Geometry: final body of the model. Coordinates: model frame, mm. Face numbers are marked on the shaded views. A direction names the side the tool comes from. Give positions to 0.01 mm unless a question says otherwise; leave off trailing zeros. Order: outer loops, then holes, each group sorted by start corner. A loop starts at its lowest first (then second) coordinate and runs counter-clockwise, first axis right, second up. Notation, with made-up numbers: M 89.25,75 L 129.25,75 A24 ccw 129.25,105 Z; hole C 18,-3 d9. An arc over 180 degrees is marked long. Use CSV: the item, a comma, the result in double quotes.
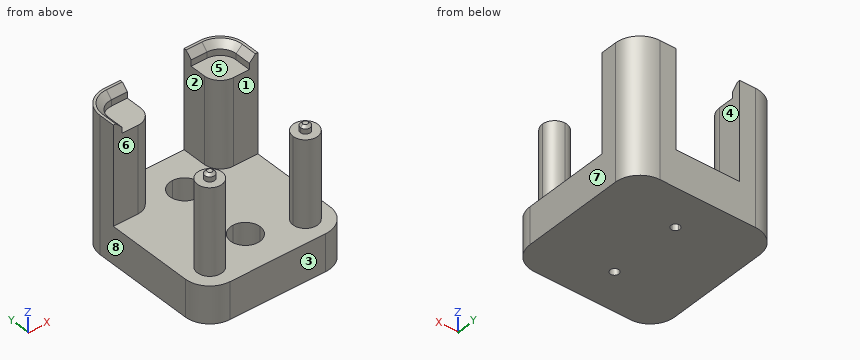
```python
from build123d import *

# Parameters (mm, degrees)
F0_W     = 26
F0_H     = 3.5
F1_DEPTH = 15
F2_DEPTH = 50
F3_DEPTH = 53
F4_DEPTH = 3
F5_DEPTH = 55
F6_SIZE  = 2.5
F7_SIZE  = 1


# Not quite as in the source:
# - a feature names something its author has since deleted; it is built from what else it names


with BuildPart() as f1:
    # F0 (on Top) → F1 (new body)
    with BuildSketch(Plane.XY):
        with Locations((0, 29.25)):
            Rectangle(F0_W, F0_H)
        with BuildLine():
            Line((29.5, -21), (29.5, 14.5))
            Line((29.5, 14.5), (26, 14.5))
            Line((26, 14.5), (19.5, 14.5))
            Line((19.5, 14.5), (19.5, 0))
            Line((19.5, 0), (19.5, -16))
            ThreePointArc((19.5, -16), (23.0355339059, -17.4644660941), (24.5, -21))
            ThreePointArc((24.5, -21), (19.5, -26), (14.5, -21))
            Line((14.5, -21), (0, -21))
            Line((0, -21), (-14.5, -21))
            ThreePointArc((-14.5, -21), (-23.0355339059, -24.5355339059), (-19.5, -16))
            Line((-19.5, -16), (-19.5, 14.5))
            Line((-19.5, 14.5), (-26, 14.5))
            Line((-26, 14.5), (-29.5, 14.5))
            Line((-29.5, 14.5), (-29.5, -21))
            ThreePointArc((-29.5, -21), (-26.5710678119, -28.0710678119), (-19.5, -31))
            Line((-19.5, -31), (19.5, -31))
            ThreePointArc((19.5, -31), (26.5710678119, -28.0710678119), (29.5, -21))
        make_face()
        with BuildLine():
            Line((19.5, 0), (19.5, 14.5))
            Line((19.5, 14.5), (5.9791303716, 14.5))
            ThreePointArc((5.9791303716, 14.5), (4.0620192023, 10.5841195668), (0, 9))
            Line((0, 9), (0, 0))
            Line((0, 0), (19.5, 0))
        make_face()
        with BuildLine():
            Line((-5.9791303716, 14.5), (-19.5, 14.5))
            Line((-19.5, 14.5), (-19.5, -16))
            ThreePointArc((-19.5, -16), (-15.9644660941, -17.4644660941), (-14.5, -21))
            Line((-14.5, -21), (0, -21))
            ThreePointArc((0, -21), (-6, -15), (0, -9))
            Line((0, -9), (0, 0))
            Line((0, 0), (0, 9))
            ThreePointArc((0, 9), (-4.0620192023, 10.5841195668), (-5.9791303716, 14.5))
        make_face()
        with BuildLine():
            Line((19.5, -16), (19.5, 0))
            Line((19.5, 0), (0, 0))
            Line((0, 0), (0, -9))
            ThreePointArc((0, -9), (4.2426406871, -10.7573593129), (6, -15))
            ThreePointArc((6, -15), (4.2426406871, -19.2426406871), (0, -21))
            Line((0, -21), (14.5, -21))
            ThreePointArc((14.5, -21), (15.9644660941, -17.4644660941), (19.5, -16))
        make_face()
        Polygon((13, 21), (13, 27.5), (-13, 27.5), (-13, 21), (0, 21), align=None)
        with BuildLine():
            Line((0, 21), (-13, 21))
            ThreePointArc((-13, 21), (-14.9038059223, 16.4038059223), (-19.5, 14.5))
            Line((-19.5, 14.5), (-5.9791303716, 14.5))
            ThreePointArc((-5.9791303716, 14.5), (-4.4158804332, 19.0620192023), (0, 21))
        make_face()
        with BuildLine():
            ThreePointArc((19.5, 14.5), (14.9038059223, 16.4038059223), (13, 21))
            Line((13, 21), (0, 21))
            ThreePointArc((0, 21), (4.2426406871, 19.2426406871), (6, 15))
            ThreePointArc((6, 15), (5.9947803225, 14.7497823241), (5.9791303716, 14.5))
            Line((5.9791303716, 14.5), (19.5, 14.5))
        make_face()
    extrude(amount=F1_DEPTH)

    # F0 (on Top) → F2 (join)
    with BuildSketch(Plane.XY):
        with BuildLine():
            ThreePointArc((-13, 21), (-14.9038059223, 25.5961940777), (-19.5, 27.5))
            ThreePointArc((-19.5, 27.5), (-24.0961940777, 25.5961940777), (-26, 21))
            ThreePointArc((-26, 21), (-24.0961940777, 16.4038059223), (-19.5, 14.5))
            Line((-19.5, 14.5), (-19.5, 21))
            Line((-19.5, 21), (-13, 21))
        make_face()
        with BuildLine():
            ThreePointArc((-19.5, 14.5), (-14.9038059223, 16.4038059223), (-13, 21))
            Line((-13, 21), (-19.5, 21))
            Line((-19.5, 21), (-19.5, 14.5))
        make_face()
        with BuildLine():
            Line((-13, 21), (-13, 27.5))
            Line((-13, 27.5), (-19.5, 27.5))
            ThreePointArc((-19.5, 27.5), (-14.9038059223, 25.5961940777), (-13, 21))
        make_face()
        with BuildLine():
            ThreePointArc((26, 21), (24.0961940777, 25.5961940777), (19.5, 27.5))
            ThreePointArc((19.5, 27.5), (14.9038059223, 25.5961940777), (13, 21))
            Line((13, 21), (19.5, 21))
            Line((19.5, 21), (19.5, 14.5))
            ThreePointArc((19.5, 14.5), (24.0961940777, 16.4038059223), (26, 21))
        make_face()
        with BuildLine():
            Line((19.5, 21), (13, 21))
            ThreePointArc((13, 21), (14.9038059223, 16.4038059223), (19.5, 14.5))
            Line((19.5, 14.5), (19.5, 21))
        make_face()
        with BuildLine():
            ThreePointArc((24.5, -21), (23.0355339059, -17.4644660941), (19.5, -16))
            Line((19.5, -16), (19.5, -19))
            ThreePointArc((19.5, -19), (20.9142135624, -19.5857864376), (21.5, -21))
            ThreePointArc((21.5, -21), (19.5, -23), (17.5, -21))
            Line((17.5, -21), (14.5, -21))
            ThreePointArc((14.5, -21), (19.5, -26), (24.5, -21))
        make_face()
        with BuildLine():
            Line((19.5, -19), (19.5, -16))
            ThreePointArc((19.5, -16), (15.9644660941, -17.4644660941), (14.5, -21))
            Line((14.5, -21), (17.5, -21))
            ThreePointArc((17.5, -21), (18.0857864376, -19.5857864376), (19.5, -19))
        make_face()
        with BuildLine():
            Line((-19.5, -19), (-19.5, -16))
            ThreePointArc((-19.5, -16), (-23.0355339059, -24.5355339059), (-14.5, -21))
            Line((-14.5, -21), (-17.5, -21))
            ThreePointArc((-17.5, -21), (-20.9142135624, -22.4142135624), (-19.5, -19))
        make_face()
        with BuildLine():
            ThreePointArc((-14.5, -21), (-15.9644660941, -17.4644660941), (-19.5, -16))
            Line((-19.5, -16), (-19.5, -19))
            ThreePointArc((-19.5, -19), (-18.0857864376, -19.5857864376), (-17.5, -21))
            Line((-17.5, -21), (-14.5, -21))
        make_face()
        with BuildLine():
            Line((19.5, 27.5), (13, 27.5))
            Line((13, 27.5), (13, 21))
            ThreePointArc((13, 21), (14.9038059223, 25.5961940777), (19.5, 27.5))
        make_face()
        with BuildLine():
            Line((19.5, 14.5), (26, 14.5))
            Line((26, 14.5), (26, 21))
            ThreePointArc((26, 21), (24.0961940777, 16.4038059223), (19.5, 14.5))
        make_face()
        with BuildLine():
            ThreePointArc((-19.5, 14.5), (-24.0961940777, 16.4038059223), (-26, 21))
            Line((-26, 21), (-26, 14.5))
            Line((-26, 14.5), (-19.5, 14.5))
        make_face()
    extrude(amount=F2_DEPTH)

    # F0 (on Top) → F3 (join)
    with BuildSketch(Plane.XY):
        with BuildLine():
            Line((-19.5, -21), (-19.5, -19))
            ThreePointArc((-19.5, -19), (-20.9142135624, -22.4142135624), (-17.5, -21))
            Line((-17.5, -21), (-19.5, -21))
        make_face()
        with BuildLine():
            ThreePointArc((-17.5, -21), (-18.0857864376, -19.5857864376), (-19.5, -19))
            Line((-19.5, -19), (-19.5, -21))
            Line((-19.5, -21), (-17.5, -21))
        make_face()
        with BuildLine():
            Line((19.5, -21), (19.5, -19))
            ThreePointArc((19.5, -19), (18.0857864376, -19.5857864376), (17.5, -21))
            Line((17.5, -21), (19.5, -21))
        make_face()
        with BuildLine():
            ThreePointArc((21.5, -21), (20.9142135624, -19.5857864376), (19.5, -19))
            Line((19.5, -19), (19.5, -21))
            Line((19.5, -21), (17.5, -21))
            ThreePointArc((17.5, -21), (19.5, -23), (21.5, -21))
        make_face()
    extrude(amount=F3_DEPTH)

    # F0 (on Top) → F4 (join)
    with BuildSketch(Plane.XY):
        with BuildLine():
            Line((-1.6770509831, 14.5), (-5.9791303716, 14.5))
            ThreePointArc((-5.9791303716, 14.5), (-4.0620192023, 10.5841195668), (0, 9))
            Line((0, 9), (0, 13.25))
            ThreePointArc((0, 13.25), (-1.0458250332, 13.59687848), (-1.6770509831, 14.5))
        make_face()
        with BuildLine():
            ThreePointArc((0, 9), (4.0620192023, 10.5841195668), (5.9791303716, 14.5))
            Line((5.9791303716, 14.5), (1.6770509831, 14.5))
            ThreePointArc((1.6770509831, 14.5), (1.0458250332, 13.59687848), (0, 13.25))
            Line((0, 13.25), (0, 9))
        make_face()
        with BuildLine():
            ThreePointArc((6, 15), (4.2426406871, 19.2426406871), (0, 21))
            ThreePointArc((0, 21), (-4.4158804332, 19.0620192023), (-5.9791303716, 14.5))
            Line((-5.9791303716, 14.5), (-1.6770509831, 14.5))
            ThreePointArc((-1.6770509831, 14.5), (-0.2526467688, 16.7316667145), (1.75, 15))
            ThreePointArc((1.75, 15), (1.7316667145, 14.7473532312), (1.6770509831, 14.5))
            Line((1.6770509831, 14.5), (5.9791303716, 14.5))
            ThreePointArc((5.9791303716, 14.5), (5.9947803225, 14.7497823241), (6, 15))
        make_face()
        with BuildLine():
            ThreePointArc((6, -15), (4.2426406871, -10.7573593129), (0, -9))
            ThreePointArc((0, -9), (-6, -15), (0, -21))
            ThreePointArc((0, -21), (4.2426406871, -19.2426406871), (6, -15))
        make_face()
        with BuildLine():
            ThreePointArc((1.75, -15), (-1.2374368671, -16.2374368671), (0, -13.25))
            ThreePointArc((0, -13.25), (1.2374368671, -13.7625631329), (1.75, -15))
        make_face(mode=Mode.SUBTRACT)
    extrude(amount=F4_DEPTH)

    # F0 (on Top) → F5 (join)
    with BuildSketch(Plane.XY):
        with BuildLine():
            ThreePointArc((29.5, 21), (26.5710678119, 28.0710678119), (19.5, 31))
            Line((19.5, 31), (13, 31))
            Line((13, 31), (13, 27.5))
            Line((13, 27.5), (19.5, 27.5))
            ThreePointArc((19.5, 27.5), (24.0961940777, 25.5961940777), (26, 21))
            Line((26, 21), (26, 14.5))
            Line((26, 14.5), (29.5, 14.5))
            Line((29.5, 14.5), (29.5, 21))
        make_face()
        with BuildLine():
            Line((-13, 27.5), (-13, 31))
            Line((-13, 31), (-19.5, 31))
            ThreePointArc((-19.5, 31), (-26.5710678119, 28.0710678119), (-29.5, 21))
            Line((-29.5, 21), (-29.5, 14.5))
            Line((-29.5, 14.5), (-26, 14.5))
            Line((-26, 14.5), (-26, 21))
            ThreePointArc((-26, 21), (-24.0961940777, 25.5961940777), (-19.5, 27.5))
            Line((-19.5, 27.5), (-13, 27.5))
        make_face()
    extrude(amount=F5_DEPTH)

    # F6
    f6_edges = [f1.edges().sort_by_distance(p)[0] for p in [
        (24.096194, 25.596194, 55),
        (16.25, 27.5, 55),
        (-16.25, 27.5, 55),
        (-24.096194, 25.596194, 55),
    ]]
    chamfer(f6_edges, length=F6_SIZE)

    # F7
    f7_edges = [f1.edges().sort_by_distance(p)[0] for p in [
        (-21.5, -21, 53),
        (21.5, -21, 53),
    ]]
    chamfer(f7_edges, length=F7_SIZE)


solid = f1.part
```
1. Section B-B, the plane z = 31.5. Return the cut outline in (x, y), plus the area to 3 significant figures.
Answer:
outline,"M -29.5,14.5 L -19.5,14.5 A6.5 ccw -13,21 L -13,31 L -19.5,31 A10 ccw -29.5,21 Z; C -19.5,-21 d10; M 13,21 A6.5 ccw 19.5,14.5 L 29.5,14.5 L 29.5,21 A10 ccw 19.5,31 L 13,31 Z; C 19.5,-21 d10"
area,"641 mm2"
2. Section A-A, the plane z = 13. Return the cut outline in (x, y).
Answer:
outline,"M -29.5,-21 A10 ccw -19.5,-31 L 19.5,-31 A10 ccw 29.5,-21 L 29.5,21 A10 ccw 19.5,31 L -19.5,31 A10 ccw -29.5,21 Z; hole C 0,-15 d12; hole C 0,15 d12"
3. Reachability of the marked faces 4, 5, 6, 7 and 8 from +Z, -Z, +X, -X, +Y, -Y: full face, straight path, thin tool, end or side. Return the list, or none.
Answer:
face 4,"+Z, +Y, -Y"
face 5,"+Z"
face 6,"+Z, +X, -X"
face 7,"+Z, -Z, +X, +Y, -Y"
face 8,"+Z, -Z, -X, +Y, -Y"
4. Section C-C, the plane x = 15.5. Return the cut outline in (y, z).
Answer:
outline,"M -31,0 L 31,0 L 31,55 L 30,55 L 27.5,52.5 L 27.5,50 L 15.88,50 L 15.88,15 L -18,15 L -18,50 L -24,50 L -24,15 L -31,15 Z"
5. Pin query (flat end, axial travel): pin 1 Ø6.5 at (x, y) = (19.5, 21.5) entering from +Z; pin 2 Ø3 at (x, y) = (0, -15) entering from -Z; pin 3 Ø5 at (x, y) = (-19.5, -22.5) entering from +Z; pin 4 Ø8 at (x, z) = (-26, 30.5) entering from -Y. Return the tip coordinate at first contact, or that it passes through.
Answer:
pin 1,"z = 50"
pin 2,"through"
pin 3,"z = 53"
pin 4,"y = -25.33"
6. Section D-D, the plane x = -10.5. Return the cut outline in (y, z).
Answer:
outline,"M -31,0 L 31,0 L 31,15 L -31,15 Z"
7. Line query: line 1 (Y direction, x = 0, z = 0.9); line 2 (X direction, y = -15, z = 2.1); line 3 (Z direction, x = 4.5, y = 1). Output: solid intervals per line, ascending.
Answer:
line 1,"-31 to -16.75, -13.25 to 13.25, 16.75 to 31"
line 2,"-29.5 to -1.75, 1.75 to 29.5"
line 3,"0 to 15"
8. Pull-direction query (Y, two-part tool) for the marked faces 1, 2 and 3; classes: +Y half, -Y half, draft (parallel to the pull), parting line (faces both ways), or undercut.
Answer:
face 1,"undercut"
face 2,"draft"
face 3,"-Y half"
